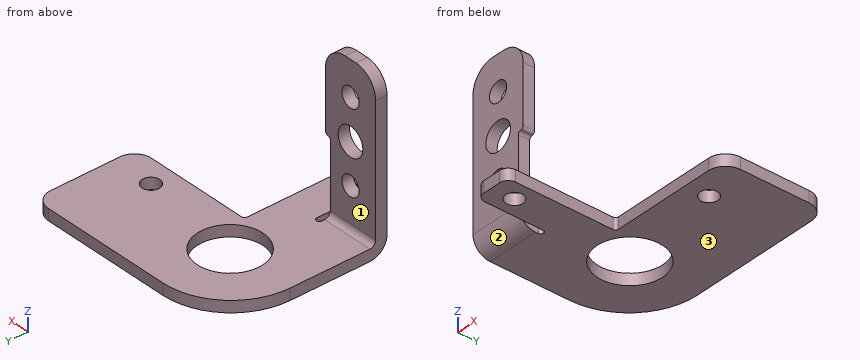
from build123d import *

# Parameters (mm, degrees)
BOSS_EXTRUDE1_DEPTH = 2
BOSS_EXTRUDE2_DEPTH = 9.2
SKETCH3_W           = 9.2
SKETCH3_H           = 2
BOSS_EXTRUDE3_DEPTH = 11.84
SKETCH4_W           = 10.2
SKETCH4_H           = 14.6
BOSS_EXTRUDE4_DEPTH = 2
FILLET1_R           = 3
FILLET2_R           = 12
SKETCH5_R           = 1.55
CUT_EXTRUDE1_DEPTH  = 60.966937557
FILLET3_R           = 1.5
FILLET4_R           = 0.5
FILLET5_R           = 0.5
FILLET6_R           = 4
FILLET7_R           = 0.5
SKETCH6_R           = 5.75
CUT_EXTRUDE2_DEPTH  = 60.966937557
SKETCH7_R           = 1.75
SKETCH7_R_2         = 2.5
CUT_EXTRUDE3_DEPTH  = 56.271634678


with BuildPart() as part:
    # Sketch1 → Boss-Extrude1 (new body)
    with BuildSketch(Plane.XY):
        Polygon((0, 0), (-38.2, 0), (-38.2, -26), (-29, -26), (-29, -25), (-28, -25), (-28, -37.2), (-21.8, -37.2), (-21.8, -18.1), (0, -18.1), align=None)
    extrude(amount=BOSS_EXTRUDE1_DEPTH)

    # Sketch2 → Boss-Extrude2 (add)
    with BuildSketch(Plane.ZY.offset(38.2)):
        with BuildLine():
            Line((0, -26), (2, -26))
            ThreePointArc((2, -26), (2.292893219, -26.707106781), (3, -27))
            Line((3, -27), (3, -29))
            ThreePointArc((3, -29), (0.878679656, -28.121320344), (0, -26))
        make_face()
    extrude(amount=-BOSS_EXTRUDE2_DEPTH)

    # Sketch3 → Boss-Extrude3 (add)
    with BuildSketch(Plane.XY.offset(3)):
        with Locations((-33.6, -28)):
            Rectangle(SKETCH3_W, SKETCH3_H)
    extrude(amount=BOSS_EXTRUDE3_DEPTH)

    # Sketch4 → Boss-Extrude4 (add)
    with BuildSketch(Plane(origin=(0, -27, 0), x_dir=(1, 0, 0), z_dir=(0, 1, 0))):
        with Locations((-33.1, -22.14)):
            Rectangle(SKETCH4_W, SKETCH4_H)
    extrude(amount=-BOSS_EXTRUDE4_DEPTH)

    # Fillet1
    fillet1_edges = [part.edges().sort_by_distance(p)[0] for p in [
        (0, -18.1, 1),
        (0, 0, 1),
    ]]
    fillet(fillet1_edges, radius=FILLET1_R)

    # Fillet2
    fillet2_edges = [part.edges().sort_by_distance(p)[0] for p in [
        (-38.2, 0, 1),
    ]]
    fillet(fillet2_edges, radius=FILLET2_R)

    # Sketch5 → Cut-Extrude1 (cut, through all)
    with BuildSketch(Plane.XY.offset(2)):
        with Locations((-7.5, -14.1)):
            Circle(SKETCH5_R)
        with Locations((-24.9, -33.2)):
            Circle(SKETCH5_R)
    extrude(amount=-CUT_EXTRUDE1_DEPTH, mode=Mode.SUBTRACT)

    # Fillet3
    fillet3_edges = [part.edges().sort_by_distance(p)[0] for p in [
        (-21.8, -37.2, 1),
        (-28, -37.2, 1),
    ]]
    fillet(fillet3_edges, radius=FILLET3_R)

    # Fillet4
    fillet4_edges = [part.edges().sort_by_distance(p)[0] for p in [
        (-28, -25, 1),
        (-29, -25, 1),
    ]]
    fillet(fillet4_edges, radius=FILLET4_R - 0.0001)  # a hair under: the kernel refuses the full size

    # Fillet5
    fillet5_edges = [part.edges().sort_by_distance(p)[0] for p in [
        (-29, -28, 14.84),
    ]]
    fillet(fillet5_edges, radius=FILLET5_R)
    fillet5_2_edges = [part.edges().sort_by_distance(p)[0] for p in [
        (-28, -28, 14.84),
    ]]
    fillet(fillet5_2_edges, radius=FILLET5_R - 0.0001)  # a hair under: the kernel refuses the full size

    # Fillet6
    fillet6_edges = [part.edges().sort_by_distance(p)[0] for p in [
        (-38.2, -28, 29.44),
        (-28, -28, 29.44),
    ]]
    fillet(fillet6_edges, radius=FILLET6_R)

    # Fillet7
    fillet7_edges = [part.edges().sort_by_distance(p)[0] for p in [
        (-21.8, -18.1, 1),
    ]]
    fillet(fillet7_edges, radius=FILLET7_R)

    # Sketch6 → Cut-Extrude2 (cut, through all)
    with BuildSketch(Plane.XY.offset(2)):
        with Locations((-26, -12)):
            Circle(SKETCH6_R)
    extrude(amount=-CUT_EXTRUDE2_DEPTH, mode=Mode.SUBTRACT)

    # Sketch7 → Cut-Extrude3 (cut, through all)
    with BuildSketch(Plane(origin=(0, -27, 0), x_dir=(1, 0, 0), z_dir=(0, 1, 0))):
        with Locations(Location((-33.1, -23.342208336, 0), (0, 0, 270))):
            Circle(SKETCH7_R)
        with Locations(Location((-33.1, -9.097791664, 0), (0, 0, 270))):
            Circle(SKETCH7_R)
        with Locations(Location((-33.1, -16.22, 0), (0, 0, 270))):
            Circle(SKETCH7_R_2)
    extrude(amount=-CUT_EXTRUDE3_DEPTH, mode=Mode.SUBTRACT)


solid = part.part
Verification items for the finished model (mm, model axes). Face numbers are marked on the shaded views. A direction names the side the tool comes from. Round coordinates to 2 decimals unless told otherwise and drop trailing zeros. Loops run counter-clockwise (first coordinate to the right, second up) from the corner with the lowest first, then second, coordinate; pieces in that order, holes last. Notation, with made-up numbers: (64.5, 34.5) - (114.5, 34.5) arc R26 cw to (114.5, 49.5) - close; hole circle Ø2 at (13.5, -3.75). An arc over 180 degrees is marked (long way). Answer in a Markdown table with one row per item. Add a question column.
Q1. Section check C-C on x = -24. Enter the section's corners in (y, z), plus the area to 3 significant figures.
Q2. Material ranges on line 1 (Y direction, x = -30.5, z = 12.75); line 2 (Y direction, x = -7.5, z = 0.85); line 3 (X direction, y = -28, z = 24.25), recorded low to high.
Q3. Section check A-A on y = -33.2. Enter the section's corners in (x, z), plus the area to 3 significant figures.
Q4. Section check B-B on z = 16.22. Enter the section's corners in (x, y).
Q5. Tool access check on the marked faces 1, 2 and 3. Record the directions out of +Z, -Z, +X, -X, +Y, -Y that give a thin tool (end or side, any length) a straight path to the whole face; none if there is none.
Q6. Gauge pin test, flat ends, axial feed: pin 1 (12 mm diameter, centred on x = -4.5, z = 9, fed in from +Y); pin 2 (2 mm diameter, centred on x = -6, y = -17, fed in from -Z); pin 3 (6 mm diameter, centred on x = -34, z = 15.5, fed in from -Y); pin 4 (11 mm diameter, centred on x = -33.5, z = 19, fed in from +Y). Record the tip position at first contact, or that the pin passes through.
Q7. Section check D-D on y = -14.1. Enter the section's corners in (x, z), plus the area to 3 significant figures.
Found:
| question | item | result |
|---|---|---|
| 1 | outline | (-37.2, 0) - (-34.46, 0) - (-34.46, 2) - (-37.2, 2) - close; (-31.94, 0) - (-17.39, 0) - (-17.39, 2) - (-31.94, 2) - close; (-6.61, 0) - (0, 0) - (0, 2) - (-6.61, 2) - close |
| 1 | area | 47.8 mm² |
| 2 | line 1 | y = -29 to -27 |
| 2 | line 2 | y = -18.1 to -15.65, -12.55 to 0 |
| 2 | line 3 | x = -38.2 to -34.6, -31.6 to -28 |
| 3 | outline | (-28, 0) - (-26.45, 0) - (-26.45, 2) - (-28, 2) - close; (-23.35, 0) - (-21.8, 0) - (-21.8, 2) - (-23.35, 2) - close |
| 3 | area | 6.20 mm² |
| 4 | outline | (-38.2, -29) - (-35.6, -29) - (-35.6, -27) - (-38.2, -27) - close; (-30.6, -29) - (-28, -29) - (-28, -27) - (-30.6, -27) - close |
| 5 | face 1 | +Z, +X, -X, +Y |
| 5 | face 2 | -Z, -X, -Y |
| 5 | face 3 | -Z, +X, -X, +Y, -Y |
| 6 | pin 1 | passes through |
| 6 | pin 2 | stops at z = 0 |
| 6 | pin 3 | stops at y = -29 |
| 6 | pin 4 | stops at y = -27 |
| 7 | outline | (-38.2, 0) - (-31.35, 0) - (-31.35, 2) - (-38.2, 2) - close; (-20.65, 0) - (-9.05, 0) - (-9.05, 2) - (-20.65, 2) - close; (-5.95, 0) - (0, 0) - (0, 2) - (-5.95, 2) - close |
| 7 | area | 48.8 mm² |
